from build123d import *

# Parameters (mm, degrees)
F0_W      = 25.4
F0_H      = 25.4
F0_W_2    = 23.368
F0_H_2    = 23.368
F1_DEPTH  = 508
F2_R      = 2.1844
F3_DEPTH  = 25.4
F4_R      = 2.1844
F5_DEPTH  = 25.4
F6_DEPTH  = 152.4
F7_R      = 2.1844
F8_DEPTH  = 25.4
F9_R      = 2.1844
F10_DEPTH = 25.4


with BuildPart() as f1:
    # F0 (on Top) → F1 (new body)
    with BuildSketch(Plane.XY):
        with Locations((12.7, -12.7)):
            Rectangle(F0_W, F0_H)
        with Locations((12.7, -12.7)):
            Rectangle(F0_W_2, F0_H_2, mode=Mode.SUBTRACT)
    extrude(amount=F1_DEPTH)

    # F2 (on face) → F3 (cut)
    with BuildSketch(Plane.XZ.offset(25.4)):
        with Locations((12.7, 12.7)):
            Circle(F2_R)
        with Locations((12.7, 38.1)):
            Circle(F2_R)
        with Locations((12.7, 241.3)):
            Circle(F2_R)
        with Locations((12.7, 215.9)):
            Circle(F2_R)
        with Locations((12.7, 190.5)):
            Circle(F2_R)
        with Locations((12.7, 165.1)):
            Circle(F2_R)
        with Locations((12.7, 139.7)):
            Circle(F2_R)
        with Locations((12.7, 114.3)):
            Circle(F2_R)
        with Locations((12.7, 88.9)):
            Circle(F2_R)
        with Locations((12.7, 63.5)):
            Circle(F2_R)
        with Locations((12.7, 266.7)):
            Circle(F2_R)
        with Locations((12.7, 292.1)):
            Circle(F2_R)
        with Locations((12.7, 317.5)):
            Circle(F2_R)
        with Locations((12.7, 342.9)):
            Circle(F2_R)
        with Locations((12.7, 368.3)):
            Circle(F2_R)
        with Locations((12.7, 393.7)):
            Circle(F2_R)
        with Locations((12.7, 419.1)):
            Circle(F2_R)
        with Locations((12.7, 444.5)):
            Circle(F2_R)
        with Locations((12.7, 469.9)):
            Circle(F2_R)
        with Locations((12.7, 495.3)):
            Circle(F2_R)
        with Locations((12.7, 520.7)):
            Circle(F2_R)
        with Locations((12.7, 546.1)):
            Circle(F2_R)
        with Locations((12.7, 571.5)):
            Circle(F2_R)
        with Locations((12.7, 596.9)):
            Circle(F2_R)
        with Locations((12.7, 622.3)):
            Circle(F2_R)
    extrude(amount=-F3_DEPTH, mode=Mode.SUBTRACT)

    # F4 (on face) → F5 (cut)
    with BuildSketch(Plane(origin=(0, 0, 0), x_dir=(0, -1, 0), z_dir=(-1, 0, 0))):
        with Locations((12.7, 12.7)):
            Circle(F4_R)
        with Locations((12.7, 38.1)):
            Circle(F4_R)
        with Locations((12.7, 63.5)):
            Circle(F4_R)
        with Locations((12.7, 88.9)):
            Circle(F4_R)
        with Locations((12.7, 114.3)):
            Circle(F4_R)
        with Locations((12.7, 139.7)):
            Circle(F4_R)
        with Locations((12.7, 165.1)):
            Circle(F4_R)
        with Locations((12.7, 190.5)):
            Circle(F4_R)
        with Locations((12.7, 215.9)):
            Circle(F4_R)
        with Locations((12.7, 241.3)):
            Circle(F4_R)
        with Locations((12.7, 266.7)):
            Circle(F4_R)
        with Locations((12.7, 292.1)):
            Circle(F4_R)
        with Locations((12.7, 317.5)):
            Circle(F4_R)
        with Locations((12.7, 342.9)):
            Circle(F4_R)
        with Locations((12.7, 368.3)):
            Circle(F4_R)
        with Locations((12.7, 393.7)):
            Circle(F4_R)
        with Locations((12.7, 419.1)):
            Circle(F4_R)
        with Locations((12.7, 444.5)):
            Circle(F4_R)
        with Locations((12.7, 546.1)):
            Circle(F4_R)
        with Locations((12.7, 520.7)):
            Circle(F4_R)
        with Locations((12.7, 495.3)):
            Circle(F4_R)
        with Locations((12.7, 469.9)):
            Circle(F4_R)
        with Locations((12.7, 571.5)):
            Circle(F4_R)
        with Locations((12.7, 596.9)):
            Circle(F4_R)
        with Locations((12.7, 622.3)):
            Circle(F4_R)
    extrude(amount=-F5_DEPTH, mode=Mode.SUBTRACT)

    # F6 (add): a face of the model
    f6_faces = [f1.faces().sort_by_distance(p)[0] for p in [
        (12.7, -0.3592102448, 0),
    ]]
    extrude(f6_faces, amount=F6_DEPTH)

    # F7 (on face) → F8 (cut)
    with BuildSketch(Plane.XZ.offset(25.4)):
        with Locations((12.7, -38.1)):
            Circle(F7_R)
        with Locations((12.7, -63.5)):
            Circle(F7_R)
        with Locations((12.7, -88.9)):
            Circle(F7_R)
        with Locations((12.7, -114.3)):
            Circle(F7_R)
        with Locations((12.7, -139.7)):
            Circle(F7_R)
    extrude(amount=-F8_DEPTH, mode=Mode.SUBTRACT)

    # F9 (on face) → F10 (cut)
    with BuildSketch(Plane(origin=(0, 0, 0), x_dir=(0, -1, 0), z_dir=(-1, 0, 0))):
        with Locations((12.7, -38.1)):
            Circle(F9_R)
        with Locations((12.7, -63.5)):
            Circle(F9_R)
        with Locations((12.7, -88.9)):
            Circle(F9_R)
        with Locations((12.7, -114.3)):
            Circle(F9_R)
        with Locations((12.7, -139.7)):
            Circle(F9_R)
    extrude(amount=-F10_DEPTH, mode=Mode.SUBTRACT)


solid = f1.part
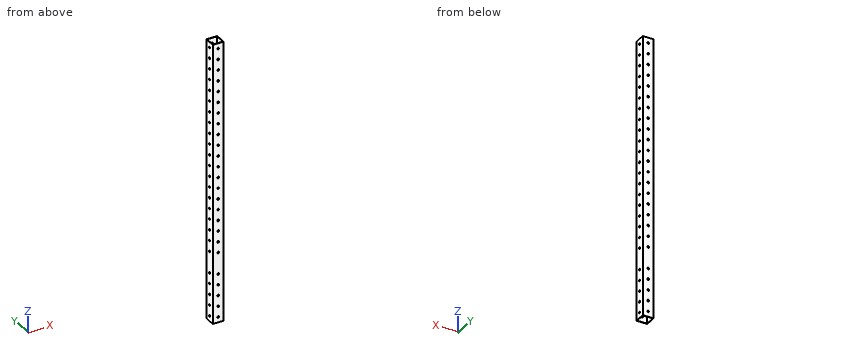
Source: CAD feature listing. Evaluate the final solid. Frame: model axes, mm. Coordinates: 2 decimals unless noted, no trailing zeros. Loops run counter-clockwise (first coordinate to the right, second up) from the corner with the lowest first, then second, coordinate; pieces in that order, holes last. Notation, with made-up numbers: (-2, 20) - (18, 20) arc R19 ccw to (18, 44) - close; hole circle Ø3 at (-39.5, -31.75). An arc over 180 degrees is marked (long way). One line per item, written item: value. Start each with the question number.
1. Section B-B (z = 411.5). Return the cut outline in (x, y).
2. Ray query, L1, parallel to Y at x = 4.5, z = 231.5; L2, parallel to X at y = -0.5, z = 495.3; L3, parallel to X at y = -11.25, z = 45. Return the intervals inside material, ascending.
3. Section A-A (y = -18.75). Return the cut outline in (x, z), and give its area (3 significant figures).
4. Contact query for a flat-ended pin moving along its axis: P1, Ø7, axis at y = -12.7, z = 393.7, coming from the -X side. Output: stop coordinate, or through.
Verdict:
1. outline: (0, -25.4) - (25.4, -25.4) - (25.4, 0) - (0, 0) - close; hole (1.02, -24.38) - (24.38, -24.38) - (24.38, -1.02) - (1.02, -1.02) - close
2. L1: y = -25.4 to -24.38, -1.02 to 0
2. L2: x = 0 to 10.52, 14.88 to 25.4
2. L3: x = 0 to 1.02, 24.38 to 25.4
3. outline: (0, -152.4) - (1.02, -152.4) - (1.02, 508) - (0, 508) - close; (24.38, -152.4) - (25.4, -152.4) - (25.4, 508) - (24.38, 508) - close
3. area: 1,340 mm2
4. P1: stops at x = 0
